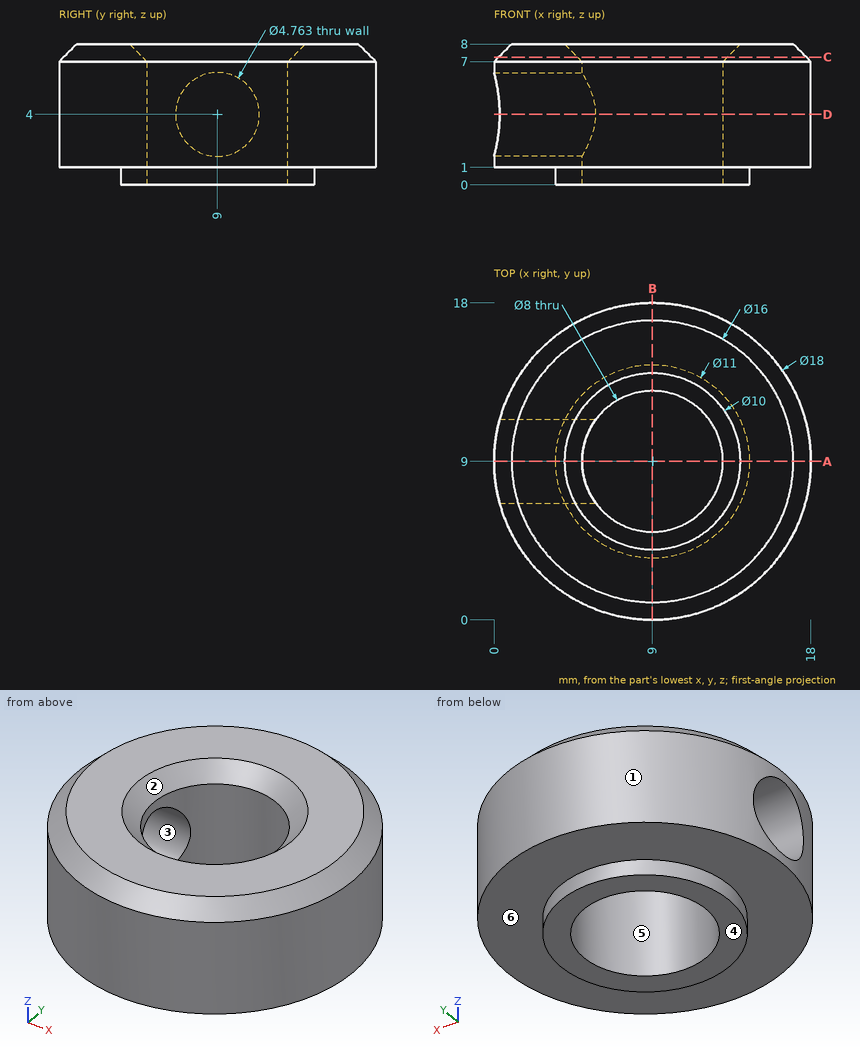
Verification items for this drawing (mm, ordinates from the low corner). A direction names the side the tool comes from. Coordinates: 2 decimals unless noted, no trailing zeros. Loops run counter-clockwise (first coordinate to the right, second up) from the corner with the lowest first, then second, coordinate; pieces in that order, holes last. Notation, with made-up numbers: (-28, -12) - (6, -12) arc R19 cw to (6, -8) - close; hole circle Ø11 at (85, -4). An arc over 180 degrees is marked (long way). Use one line per item in the form item = value. Start each with the question number.
Item 1: Mould release check, pull along Y, two halves, no side actions. Record for the marked faces 1, 2, 3 and 4: +Y half, -Y half, draft (parallel to the pull), parting line (faces both ways), or undercut.
Item 2: Section check A-A, the plane y = 9. Enter the section's corners in (x, z).
Item 3: Section check D-D, the plane z = 4. Enter the section's corners in (x, y), and give its area (3 significant figures).
Item 4: Thickness scan on probe 1 along Y at (x, z) = (9, 5.75); probe 2 along Z at (x, y) = (14.5, 8.25); probe 3 along Y at (x, z) = (10.25, 0.75) (1 decimal). Record the ranges inside material, lowest first.
Item 5: Tool access check on the marked faces 5 and 6. Record the directions out of +Z, -Z, +X, -X, +Y, -Y that give a thin tool (end or side, any length) a straight path to the whole face; none if there is none.
Item 6: Section check B-B, the plane x = 9. Enter the section's corners in (y, z), and give its area (3 significant figures).
Item 7: Gauge pin test, flat ends, axial feed: pin 1 (1 mm diameter, centred on x = 7, z = 5.5, fed in from +Y); pin 2 (4 mm diameter, centred on x = 4, z = 1.5, fed in from -Y) (1 decimal); pin 3 (4 mm diameter, centred on y = 10.5, z = 4.5, fed in from -X). Record the tip position at first contact, or that the pin passes through.
Item 8: Section check C-C, the plane z = 7.25. Enter the section's corners in (x, y), and give its area (3 significant figures).
Computed:
q1.face_1 = parting line
q1.face_2 = undercut
q1.face_3 = undercut
q1.face_4 = draft
q2.outline = (0, 1) - (3.5, 1) - (3.5, 0) - (5, 0) - (5, 1.62) - (0, 1.62) - close; (0, 6.38) - (5, 6.38) - (5, 7) - (4, 8) - (1, 8) - (0, 7) - close; (13, 0) - (14.5, 0) - (14.5, 1) - (18, 1) - (18, 7) - (17, 8) - (14, 8) - (13, 7) - close
q3.outline = (0.32, 6.62) arc R9 ccw (long way) to (0.32, 11.38) - (5.79, 11.38) arc R4 cw (long way) to (5.79, 6.62) - close
q3.area = 180 mm2
q4.probe_1 = 0 to 5, 13 to 18
q4.probe_2 = 1 to 8
q4.probe_3 = 3.6 to 5.2, 12.8 to 14.4
q5.face_5 = +Z, -Z
q5.face_6 = -Z
q6.outline = (0, 1) - (3.5, 1) - (3.5, 0) - (5, 0) - (5, 7) - (4, 8) - (1, 8) - (0, 7) - close; (13, 0) - (14.5, 0) - (14.5, 1) - (18, 1) - (18, 7) - (17, 8) - (14, 8) - (13, 7) - close
q6.area = 71.0 mm2
q7.pin_1 = 17.87
q7.pin_2 = 0.5
q7.pin_3 = 0.02
q8.outline = circle Ø17.5 at (9, 9); hole circle Ø8.5 at (9, 9)
q8.area = 184 mm2
